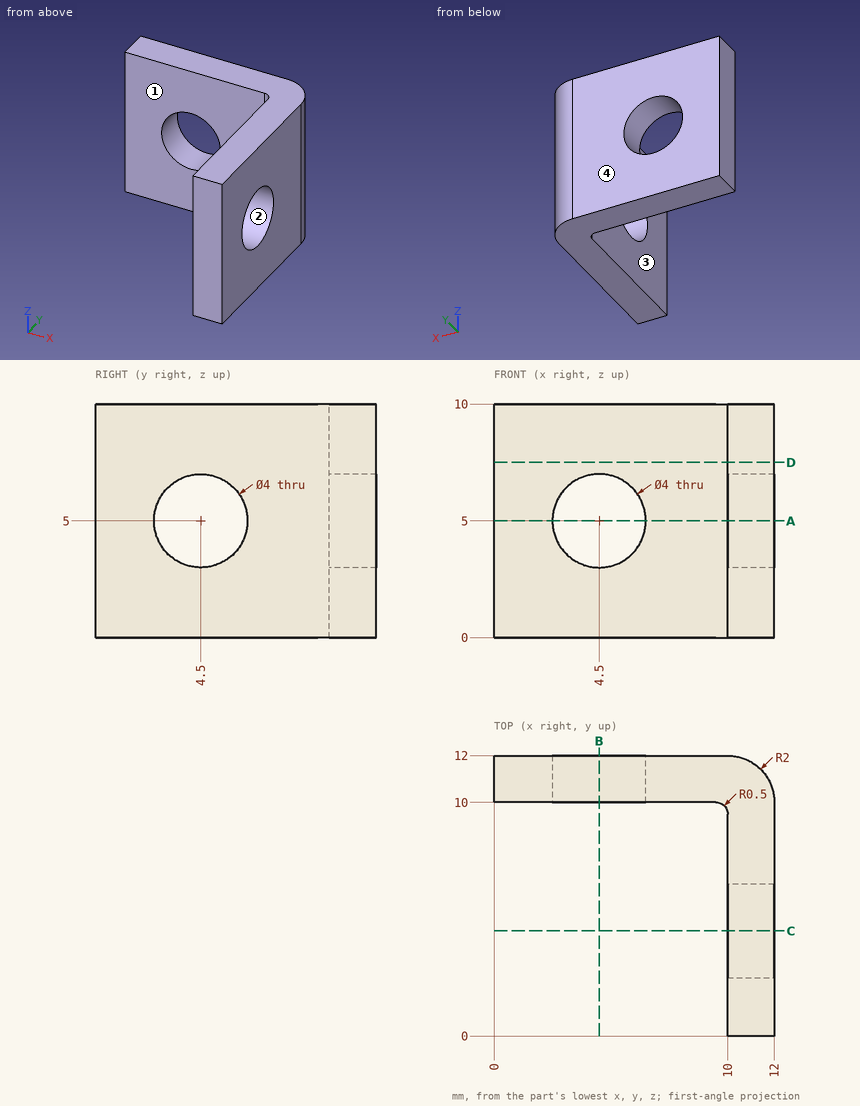
Study the drawing (mm; zero at the part's minimum x, y, z) and answer. Round coordinates to 2 decimals unless told otherwise and drop trailing zeros. Write each loop counter-clockwise with the first axis right and the second up, starting at its lowest first coordinate (ties: lowest second). Pieces come first, ordered by that corner, then holes.
Q1. A flat-ended cylindrical pin translates along its axis: P1, Ø5, axis at y = 4.5, z = 5, coming from the -X side. Find the tip coordinate at first contact, or state that the pin passes through.
Values:
P1: stops at x = 10
Q2. Find section B-B on x = 4.5. Determine the outline of the cut face in (y, z).
Values:
outline: (10, 0) - (12, 0) - (12, 3) - (10, 3) - close; (10, 7) - (12, 7) - (12, 10) - (10, 10) - close
Q3. Find section A-A on z = 5. Determine the outline of the cut face in (x, y), and give its area (3 significant figures).
Values:
outline: (0, 10) - (2.5, 10) - (2.5, 12) - (0, 12) - close; (6.5, 10) - (9.5, 10) arc R0.5 cw to (10, 9.5) - (10, 6.5) - (12, 6.5) - (12, 10) arc R2 ccw to (10, 12) - (6.5, 12) - close; (10, 0) - (12, 0) - (12, 2.5) - (10, 2.5) - close
area: 27.2 mm2
Q4. Straight lines are drawn through the part: line 1 (Z direction, x = 10.45, y = 4.5); line 2 (Y direction, x = 1, z = 4). For each, find the intervals that lie inside material, in ascending order.
Values:
line 1: z = 0 to 3, 7 to 10
line 2: y = 10 to 12
Q5. The mould has two halves that part along Y. Classify the marked faces 1, 2, 3 and 4: released by +Y, released by -Y, zero draft, split by the parting line, or undercut.
Values:
face 1: released by -Y
face 2: undercut
face 3: zero draft
face 4: released by +Y
Q6. Find section D-D on z = 7.5. Determine the outline of the cut face in (x, y), and give its area (3 significant figures).
Values:
outline: (0, 10) - (9.5, 10) arc R0.5 cw to (10, 9.5) - (10, 0) - (12, 0) - (12, 10) arc R2 ccw to (10, 12) - (0, 12) - close
area: 43.2 mm2
